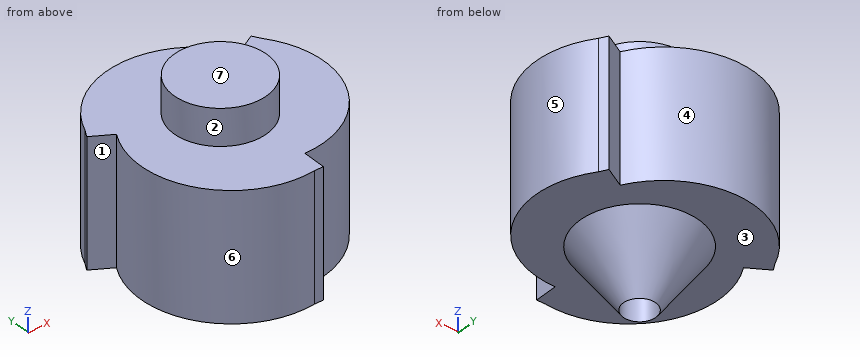
from build123d import *

# Parameters (mm, degrees)
SALIENTE_EXTRUIR1_DEPTH = 18
SALIENTE_EXTRUIR2_START = 1.5
CROQUIS2_R              = 2.7
SALIENTE_EXTRUIR2_DEPTH = 1.5
SALIENTE_EXTRUIR3_DEPTH = 1.5
CROQUIS6_W              = 5.4
CROQUIS6_H              = 1.181933233
SALIENTE_EXTRUIR7_DEPTH = 10
CROQUIS7_W              = 5.4
CROQUIS7_H              = 10
CORTAR_EXTRUIR2_DEPTH   = 16.5


with BuildPart() as part:
    # Croquis1 → Saliente-Extruir1 (new body)
    with BuildSketch(Plane.XY):
        with BuildLine():
            Line((-54.535099114, 31.482780649), (-55.25791247, 32.775048384))
            Line((-55.25791247, 32.775048384), (-58.679569293, 30.903614553))
            ThreePointArc((-58.679569293, 30.903614553), (-72.555259572, 38.768368337), (-85.712228427, 29.752642999))
            Line((-85.712228427, 29.752642999), (-86.469958437, 28.480534403))
            Line((-86.469958437, 28.480534403), (-83.138420786, 26.453009587))
            ThreePointArc((-83.138420786, 26.453009587), (-83.011652218, 10.503932418), (-68.625320614, 3.617525822))
            Line((-68.625320614, 3.617525822), (-67.144777249, 3.597366682))
            Line((-67.144777249, 3.597366682), (-67.054658077, 7.49632533))
            ThreePointArc((-67.054658077, 7.49632533), (-53.305736365, 15.580648714), (-54.535099114, 31.482780649))
        make_face()
        with BuildLine():
            Line((-69.624216052, 5.117649823), (-68.624216052, 5.117649823))
            Line((-68.624216052, 5.117649823), (-68.624216052, 9.117649823))
            ThreePointArc((-68.624216052, 9.117649823), (-55.305921191, 15.218525867), (-55.334796889, 29.867649823))
            Line((-55.334796889, 29.867649823), (-55.834796889, 30.733675227))
            Line((-55.834796889, 30.733675227), (-59.298898504, 28.733675227))
            ThreePointArc((-59.298898504, 28.733675227), (-71.241559574, 37.21721889), (-83.913635214, 29.867649823))
            Line((-83.913635214, 29.867649823), (-84.413635214, 29.001624419))
            Line((-84.413635214, 29.001624419), (-80.949533599, 27.001624419))
            ThreePointArc((-80.949533599, 27.001624419), (-82.325167391, 12.417204713), (-69.624216052, 5.117649823))
        make_face(mode=Mode.SUBTRACT)
    extrude(amount=SALIENTE_EXTRUIR1_DEPTH)

    # Croquis2 → Saliente-Extruir2 (add)
    with BuildSketch(Plane(origin=(0, 0, 0), x_dir=(-1, 0, 0), z_dir=(0, 0, -1)).offset(SALIENTE_EXTRUIR2_START)):
        with BuildLine():
            Line((67.054658077, 7.49632533), (67.144777249, 3.597366682))
            Line((67.144777249, 3.597366682), (68.625320614, 3.617525822))
            ThreePointArc((68.625320614, 3.617525822), (83.011652218, 10.503932418), (83.138420786, 26.453009587))
            Line((83.138420786, 26.453009587), (86.469958437, 28.480534403))
            Line((86.469958437, 28.480534403), (85.712228427, 29.752642999))
            ThreePointArc((85.712228427, 29.752642999), (72.555259572, 38.768368337), (58.679569293, 30.903614553))
            Line((58.679569293, 30.903614553), (55.25791247, 32.775048384))
            Line((55.25791247, 32.775048384), (54.535099114, 31.482780649))
            ThreePointArc((54.535099114, 31.482780649), (53.305736365, 15.580648714), (67.054658077, 7.49632533))
        make_face()
        with Locations((69.624216052, 21.617649823)):
            Circle(CROQUIS2_R, mode=Mode.SUBTRACT)
    extrude(amount=-SALIENTE_EXTRUIR2_DEPTH)

    # Croquis3 → Saliente-Extruir3 (add)
    with BuildSketch(Plane.XY.offset(18)):
        with BuildLine():
            Line((-67.144777249, 3.597366682), (-67.054658077, 7.49632533))
            ThreePointArc((-67.054658077, 7.49632533), (-53.305736365, 15.580648714), (-54.535099114, 31.482780649))
            Line((-54.535099114, 31.482780649), (-55.25791247, 32.775048384))
            Line((-55.25791247, 32.775048384), (-58.679569293, 30.903614553))
            ThreePointArc((-58.679569293, 30.903614553), (-72.555259572, 38.768368337), (-85.712228427, 29.752642999))
            Line((-85.712228427, 29.752642999), (-86.469958437, 28.480534403))
            Line((-86.469958437, 28.480534403), (-83.138420786, 26.453009587))
            ThreePointArc((-83.138420786, 26.453009587), (-83.011652218, 10.503932418), (-68.625320614, 3.617525822))
            Line((-68.625320614, 3.617525822), (-67.144777249, 3.597366682))
        make_face()
    extrude(amount=SALIENTE_EXTRUIR3_DEPTH)

    # Croquis6 → Saliente-Extruir7 (add)
    with BuildSketch(Plane(origin=(0, 0, -1.5), x_dir=(-1, 0, 0), z_dir=(0, 0, -1))):
        with Locations((69.624216052, 21.026683207)):
            Rectangle(CROQUIS6_W, CROQUIS6_H)
    extrude(amount=SALIENTE_EXTRUIR7_DEPTH)

    # Croquis7 → Cortar-Extruir2 (cut)
    with BuildSketch(Plane(origin=(0, 21.617649823, 0), x_dir=(1, 0, 0), z_dir=(0, 1, 0))):
        with Locations((-69.624216052, 6.5)):
            Rectangle(CROQUIS7_W, CROQUIS7_H)
    extrude(amount=-CORTAR_EXTRUIR2_DEPTH, mode=Mode.SUBTRACT)

    # Croquis8 → Revolución1 (revolve)
    with BuildSketch(Plane(origin=(0, 21.617649823, 0), x_dir=(1, 0, 0), z_dir=(0, 1, 0)), mode=Mode.PRIVATE) as revoluci_n1_sk:
        Polygon((-72.324216052, 1.5), (-79.486781688, 1.5), (-72.324216052, 11.5), align=None)
        Polygon((-72.324216052, -19.5), (-69.624216052, -19.5), (-69.624216052, -25.5), (-72.324216052, -25.5), (-77.324216052, -25.5), (-77.324216052, -19.5), align=None)
    revolve(revoluci_n1_sk.sketch.rotate(Axis((-69.624216052, 21.617649823, 19.5), (0, 0, 1)), 180), axis=Axis((-69.624216052, 21.617649823, 19.5), (0, 0, 1)))


solid = part.part
Build history of the part. All positions in model axes, mm. Face numbers are marked on the shaded views. A direction names the side the tool comes from. Round coordinates to 2 decimals unless told otherwise and drop trailing zeros. Loops run counter-clockwise (first coordinate to the right, second up) from the corner with the lowest first, then second, coordinate; pieces in that order, holes last. Notation, with made-up numbers: (87.25, 1.25) -> (107.25, 1.25) arc R29 cw to (107.25, 34.25) -> close; hole circle Ø11 at (-1.75, 77.25). An arc over 180 degrees is marked (long way). Answer in a Markdown table with one row per item.
Item 1: Saw through at D-D (x = -82.5). Write the cut outline in (y, z), and give its area (3 significant figures).
Answers below:
| item | result |
|---|---|
| outline | (9.75, -1.5) -> (34.43, -1.5) -> (34.43, 19.5) -> (9.75, 19.5) -> close; hole (12.77, 0) -> (24.51, 0) -> (24.51, 18) -> (12.77, 18) -> close; hole (27.9, 0) -> (32.07, 0) -> (32.07, 18) -> (27.9, 18) -> close |
| area | 232 mm² |
Item 2: Which spindle directions (+Z, -Z, +X, -X, +Y, -Y) get a long thin tool onto all of the face, cutting with end or side? Do the marked faces 1, 2, 3 and 4. Say none if no direction does.
Answers below:
| item | result |
|---|---|
| face 1 | +Z, -Z, -X |
| face 2 | +Z |
| face 3 | -Z |
| face 4 | +Z, -Z, +Y |
Item 3: Saw through at C-C (z = 18.5). Write the cut outline in (x, y), and give its area (3 significant figures).
Answers below:
| item | result |
|---|---|
| outline | (-86.47, 28.48) -> (-83.14, 26.45) arc R15.06 ccw to (-68.63, 3.62) -> (-67.14, 3.6) -> (-67.05, 7.5) arc R15.06 ccw to (-54.54, 31.48) -> (-55.26, 32.78) -> (-58.68, 30.9) arc R15.06 ccw to (-85.71, 29.75) -> close |
| area | 906 mm² |
Item 4: Pin check, flat tips, straight feed: pin 1 (10.5 mm diameter, centred on x = -76.5, y = 26, fed in from -Z); pin 2 (5 mm diameter, centred on x = -55.5, z = 16.5, fed in from -Y); pin 3 (1 mm diameter, centred on y = 29.5, z = 7, fed in from -X). Stop position of each tip, or through.
Answers below:
| item | result |
|---|---|
| pin 1 | stops at z = -11.22 |
| pin 2 | stops at y = 10.23 |
| pin 3 | stops at x = -86.16 |
Item 5: Saw through at A-A (z = 10). Write the cut outline in (x, y).
Answers below:
| item | result |
|---|---|
| outline | (-86.47, 28.48) -> (-83.14, 26.45) arc R15.06 ccw to (-68.63, 3.62) -> (-67.14, 3.6) -> (-67.05, 7.5) arc R15.06 ccw to (-54.54, 31.48) -> (-55.26, 32.78) -> (-58.68, 30.9) arc R15.06 ccw to (-85.71, 29.75) -> close; hole (-84.41, 29) -> (-80.95, 27) arc R13.54 ccw to (-69.62, 5.12) -> (-68.62, 5.12) -> (-68.62, 9.12) arc R13.54 ccw to (-55.33, 29.87) -> (-55.83, 30.73) -> (-59.3, 28.73) arc R13.54 ccw to (-83.91, 29.87) -> close |
Item 6: Saw through at B-B (y = 10.5). Write the cut outline in (x, z).
Answers below:
| item | result |
|---|---|
| outline | (-83.01, -1.5) -> (-57.62, -1.5) -> (-57.62, 19.5) -> (-83.01, 19.5) -> close; hole (-81.12, 0) -> (-60.48, 0) -> (-60.48, 18) -> (-81.12, 18) -> close |
Item 7: Mould opens along Y. For the marked faces 5, 6 and 7 say: +Y half, -Y half, draft (parallel to the pull), parting line (faces both ways), or undercut.
Answers below:
| item | result |
|---|---|
| face 5 | parting line |
| face 6 | undercut |
| face 7 | draft |
Item 8: Drill centre lines: L1, parallel to Z at x = -81.5, y = 14.5; L2, parallel to X at y = 29.5, z = 14.5; L3, parallel to X at y = 21.5, z = 22.5. Where is each one in solid material? Low to high. Write a range as [from, to].
Answers below:
| item | result |
|---|---|
| L1 | z = [-1.5, 0], [18, 19.5] |
| L2 | x = [-85.86, -84.13], [-59.63, -57.97], [-55.11, -53.3] |
| L3 | x = [-77.32, -61.93] |
